Verification items for the finished model (mm, model axes). Face numbers are marked on the shaded views. A direction names the side the tool comes from. Round coordinates to 2 decimals unless told otherwise and drop trailing zeros. Write each loop counter-clockwise with the first axis right and the second up, starting at its lowest first coordinate (ties: lowest second). Pieces come first, ordered by that corner, then holes.
from build123d import *

# Parameters (mm, degrees)
F1_DEPTH = 10
F2_T     = -1
F3_R     = 10.1798341208
F3_R_2   = 10.6098641694
F4_DEPTH = 1.001


with BuildPart() as f1:
    # F0 (on Top) → F1 (new body)
    with BuildSketch(Plane.XY):
        with BuildLine():
            Line((25.9413104504, 10.6388526037), (25.9413104504, 28.418853879))
            ThreePointArc((25.9413104504, 28.418853879), (-0.6152572854, 49.3227077034), (-27.3986887187, 28.7103280425))
            Line((-27.3986887187, 28.7103280425), (-27.3986887187, 9.7644263878))
            Line((-27.3986887187, 9.7644263878), (-29.000794515, 7.9723494127))
            Line((-29.000794515, 7.9723494127), (-30.7569466531, 7.9723494127))
            Line((-30.7569466531, 7.9723494127), (-33.2814157009, 9.1797038913))
            Line((-33.2814157009, 9.1797038913), (-35.9156429768, 10.8260978013))
            Line((-35.9156429768, 10.8260978013), (-38.659632206, 10.9358569607))
            Line((-38.659632206, 10.9358569607), (-41.1841012537, 9.289463982))
            Line((-41.1841012537, 9.289463982), (-41.1841012537, 6.216196809))
            Line((-41.1841012537, 6.216196809), (-35.8058847487, 2.4843721185))
            Line((-35.8058847487, 2.4843721185), (-29.0309265256, 0))
            Line((-29.0309265256, 0), (-28.1227175146, -2.8938457835))
            Line((-28.1227175146, -2.8938457835), (-29.0309265256, -5.4257945158))
            Line((-29.0309265256, -5.4257945158), (-32.3780551553, -10.902912356))
            Line((-32.3780551553, -10.902912356), (-35.7251800597, -14.6557530388))
            Line((-35.7251800597, -14.6557530388), (-39.3765941262, -18.3071661741))
            Line((-39.3765941262, -18.3071661741), (-42.9265759885, -20.944295451))
            Line((-42.9265759885, -20.944295451), (-46.0708513856, -22.5671455264))
            Line((-46.0708513856, -22.5671455264), (-49.9251186848, -22.5671455264))
            Line((-49.9251186848, -22.5671455264), (-49.9251186848, -24.2914240807))
            Line((-49.9251186848, -24.2914240807), (-48.5051237047, -25.7114171982))
            Line((-48.5051237047, -25.7114171982), (-44.6508564055, -27.4356938899))
            Line((-44.6508564055, -27.4356938899), (-36.3175208918, -29.5778558365))
            Line((-36.3175208918, -29.5778558365), (-35.3194698691, -36.5642234683))
            Line((-35.3194698691, -36.5642234683), (-30.3494930267, -35.8542278409))
            Line((-30.3494930267, -35.8542278409), (-19.9023969471, -35.8542278409))
            Line((-19.9023969471, -35.8542278409), (-13.0052855238, -40.2156375349))
            Line((-13.0052855238, -40.2156375349), (-5.9053180739, -44.9333089781))
            Line((-5.9053180739, -44.9333089781), (4.4327859365, -44.9333089781))
            Line((4.4327859365, -44.9333089781), (11.2596079707, -40.6216345727))
            Line((11.2596079707, -40.6216345727), (16.2748470902, -37.4541170895))
            Line((16.2748470902, -37.4541170895), (22.0819637179, -34.6825383604))
            Line((22.0819637179, -34.6825383604), (27.3611601442, -34.6825383604))
            Line((27.3611601442, -34.6825383604), (29.5388307422, -35.6723889709))
            Line((29.5388307422, -35.6723889709), (33.9104868472, -35.6723889709))
            Line((33.9104868472, -35.6723889709), (35.3459455073, -29.2053706944))
            Line((35.3459455073, -29.2053706944), (41.483014822, -27.8855711222))
            Line((41.483014822, -27.8855711222), (45.9846592715, -26.8396986936))
            Line((45.9846592715, -26.8396986936), (48.0585619807, -25.0806845725))
            Line((48.0585619807, -25.0806845725), (48.0585619807, -22.2740583122))
            Line((48.0585619807, -22.2740583122), (43.8938885927, -21.0065506399))
            Line((43.8938885927, -21.0065506399), (39.72921893, -19.1958248615))
            Line((39.72921893, -19.1958248615), (35.9230749309, -16.3158885314))
            Line((35.9230749309, -16.3158885314), (31.6239426274, -11.2471502964))
            Line((31.6239426274, -11.2471502964), (28.0989827636, -7.0911723973))
            Line((28.0989827636, -7.0911723973), (25.6186239421, -4.1667940095))
            Line((25.6186239421, -4.1667940095), (25.6186239421, 0))
            Line((25.6186239421, 0), (29.3620377779, 3.1750369817))
            Line((29.3620377779, 3.1750369817), (33.1457033753, 4.6643526293))
            Line((33.1457033753, 4.6643526293), (35.9230749309, 5.8316537179))
            Line((35.9230749309, 5.8316537179), (36.8488691747, 6.5561858937))
            Line((36.8488691747, 6.5561858937), (37.4928973615, 8.005249314))
            Line((37.4928973615, 8.005249314), (36.8488691747, 9.2530548573))
            Line((36.8488691747, 9.2530548573), (33.9104868472, 10.6388526037))
            Line((33.9104868472, 10.6388526037), (27.1884426475, 8.9310398325))
            Line((27.1884426475, 8.9310398325), (25.9413104504, 10.6388526037))
        make_face()
    extrude(amount=F1_DEPTH)

    # F2
    f2_openings = [f1.faces().sort_by_distance(p)[0] for p in [
        (-0.960702, -0.889332, 10),
    ]]
    offset(amount=F2_T, openings=f2_openings, kind=Kind.INTERSECTION)

    # F3 (on face) → F4 (cut, through all)
    with BuildSketch(Plane.XY.offset(1)):
        with Locations((-0.76559461, 21.8108601041)):
            Circle(F3_R)
        with Locations((0, -18.508689478)):
            Circle(F3_R_2)
    extrude(amount=-F4_DEPTH, mode=Mode.SUBTRACT)


solid = f1.part
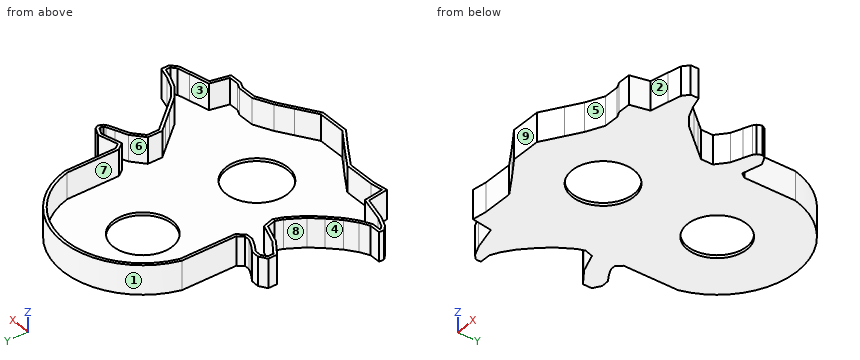
Q1. Material ranges on line 1 along Y through (x, z) = (35.5, 1.75); line 2 along X through (y, z) = (13.5, 9); line 3 along Z through (x, y) = (-18.5, -13.5), recorded low to high.
Recorded:
line 1: y = -29.17 to -28.15, -17.25 to -15.82, 5.65 to 6.77, 8.78 to 9.89
line 2: x = -27.4 to -26.4, 24.94 to 25.94
line 3: z = 0 to 1
Q2. Sectioned sample at A-A (x = 0). Enter the section's corners in (y, z), plus the area to 3 significant figures.
Recorded:
outline: (-44.93, 0) - (-29.12, 0) - (-29.12, 1) - (-43.93, 1) - (-43.93, 10) - (-44.93, 10) - close; (-7.9, 0) - (11.66, 0) - (11.66, 1) - (-7.9, 1) - close; (31.96, 0) - (49.31, 0) - (49.31, 10) - (48.31, 10) - (48.31, 1) - (31.96, 1) - close
area: 70.7 mm2
Q3. Release check for a two-part mould opening along X. For the marked faces 6, 7, 8 and 9 record: released by +X, released by -X, zero draft, split by the parting line, or undercut.
Recorded:
face 6: undercut
face 7: undercut
face 8: released by -X
face 9: zero draft
Q4. Depth check by flat-ended pin: P1, Ø4, axis at x = -13.5, z = 5.5, coming from the +Y side; P2, Ø2.5, axis at x = -47.5, z = 6.5, coming from the -Y side; P3, Ø1.9, axis at x = -49, z = 6.5, coming from the +Y side. Enter the tip coordinate at first touch or a pass-through.
Recorded:
P1: stops at y = 47.14
P2: stops at y = -26.72
P3: stops at y = -22.57
Q5. Sectioned sample at B-B (y = 43). Enter the section's corners in (x, z).
Recorded:
outline: (-18.31, 0) - (16.78, 0) - (16.78, 10) - (15.17, 10) - (15.17, 1) - (-16.7, 1) - (-16.7, 10) - (-18.31, 10) - close
Q6. Tool access check on the marked faces 1, 2, 3, 4 and 5. Record the directions out of +Z, -Z, +X, -X, +Y, -Y that give a thin tool (end or side, any length) a straight path to the whole face; none if there is none.
Recorded:
face 1: +Z, -Z, +Y
face 2: +Z, -Z, +X, -Y
face 3: +Z
face 4: +Z, -Z, -X
face 5: +Z, -Z, -Y
